Design review of the part built by this model. Coordinates are the model's own, in mm. Face numbers are marked on the shaded views. Coordinates: 2 decimals unless noted, no trailing zeros.
Q1. To check wall thickness, follow probe 1 along Y at (x, z) = (0, 6.5); probe 2 along Z at (x, y) = (63, -1); probe 3 along Z at (x, y) = (71, -1). State the ranges of each line that lie inside material, in increasing order.
Q2. Clearance check with flat-ended pins moving along their axes: pin 1 Ø8 at (x, z) = (29, 38.5) entering from -Y; pin 2 Ø6 at (x, z) = (17.5, 33) entering from -Y; pin 3 Ø4 at (x, y) = (13.5, 6.5) entering from +Z. State where each tip first meets the part, or that it passes through.
Q3. The part is to be moulded in two halves that separate along Y. For the marked faces 1 and 2, say which applies: +Y half, -Y half, draft (parallel to the pull), parting line (faces both ways), or undercut.
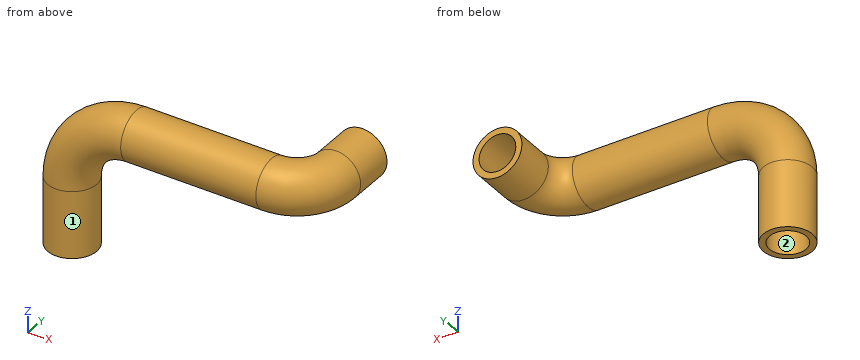
from build123d import *

# Parameters (mm, degrees)
SWEEP1_PROFILE_R                           = 8
HOLLOW_TUBE_OD_AND_WALL_PROVISIONAL_PROF_R = 6


with BuildPart() as part:
    # Sweep1: sweep along a curve in space
    with BuildLine() as sweep1_path:
        Line((0, 0, 0), (0, 0, 21.930000411))
        ThreePointArc((0, 0, 21.930000411), (6.171260145, 0, 36.828740145), (21.07, 0, 43))
        Line((21.07, 0, 43), (65.259998661, 0, 43))
        ThreePointArc((65.259998661, 0, 43), (74.268539526, 3.731459526, 43), (78, 12.74, 43))
        Line((78, 12.74, 43), (78, 26, 43))
    # Sweep1 profile (on start of the path) → Sweep1 (sweep)
    with BuildSketch(Plane.XY):
        Circle(SWEEP1_PROFILE_R)
    sweep(path=sweep1_path.line)

    # Hollow_tube_OD_and_wall_PROVISIONAL: sweep along a curve in space
    with BuildLine() as hollow_tube_od_and_wall_provisional_path:
        Line((0, 0, 0), (0, 0, 21.930000411))
        ThreePointArc((0, 0, 21.930000411), (6.171260145, 0, 36.828740145), (21.07, 0, 43))
        Line((21.07, 0, 43), (65.259998661, 0, 43))
        ThreePointArc((65.259998661, 0, 43), (74.268539526, 3.731459526, 43), (78, 12.74, 43))
        Line((78, 12.74, 43), (78, 26, 43))
    # Hollow_tube_OD_and_wall_PROVISIONAL prof (on start of the path) → Hollow_tube_OD_and_wall_PROVISIONAL (sweep, cut)
    with BuildSketch(Plane.XY):
        Circle(HOLLOW_TUBE_OD_AND_WALL_PROVISIONAL_PROF_R)
    sweep(path=hollow_tube_od_and_wall_provisional_path.line, mode=Mode.SUBTRACT)


solid = part.part
Here are the results:
1. probe 1: y = -8 to -6, 6 to 8
1. probe 2: z = 35.06 to 37.08, 48.92 to 50.94
1. probe 3: z = 35.29 to 37.4, 48.6 to 50.71
2. pin 1: stops at y = -7.98
2. pin 2: stops at y = -4.75
2. pin 3: stops at z = 48.66
3. face 1: parting line
3. face 2: undercut
